Can you work these out from the drawing? Everything is in mm from the part's minimum corner. A direction names the side the tool comes from. Give positions to 0.01 mm unless a question says otherwise; leave off trailing zeros. Order: outer loops, then holes, each group sorted by start corner. A loop starts at its lowest first (then second) coordinate and runs counter-clockwise, first axis right, second up. Notation, with made-up numbers: (-28, 19) - (11, 19) arc R23 ccw to (11, 29) - close; hole circle Ø5 at (82.5, 30.5). An arc over 180 degrees is marked (long way). Answer as a JSON object with one key per item and string values.
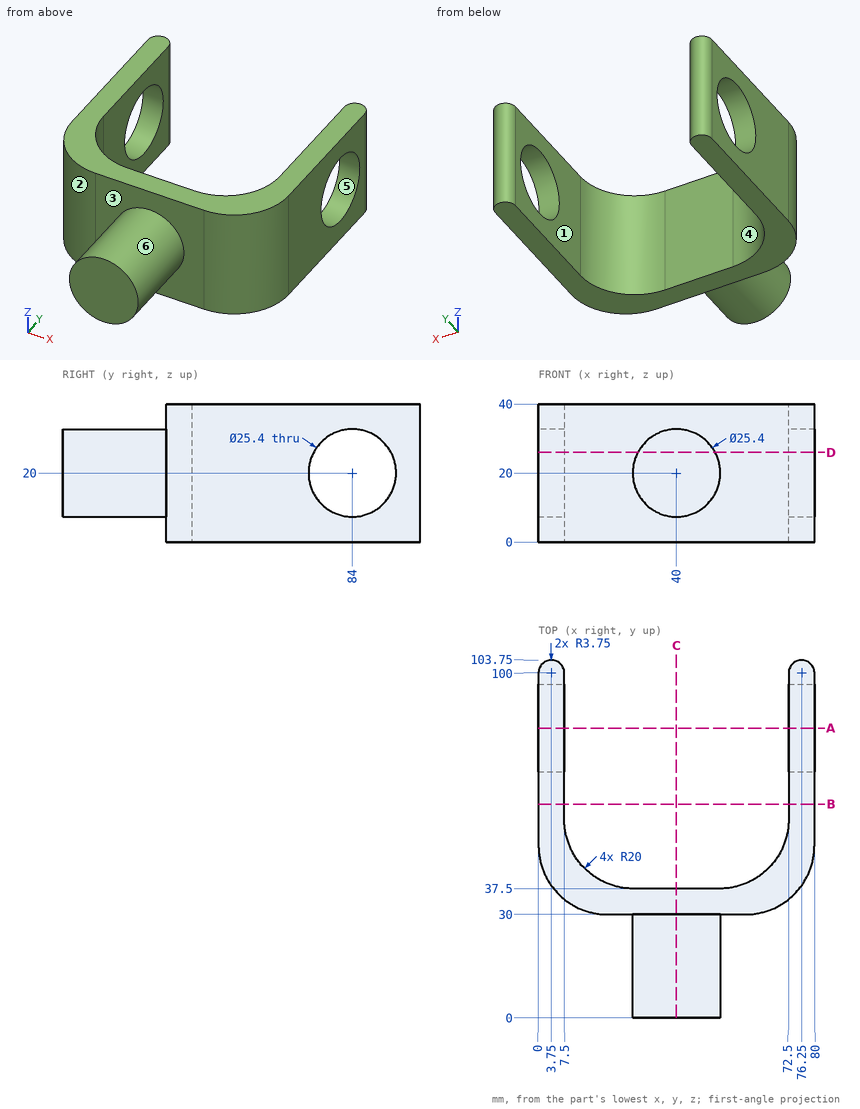
Q1. I'm going to push flat-ended pins straight in: pin 1 Ø4 at (x, z) = (58.5, 26) entering from +Y; pin 2 Ø5 at (x, z) = (59, 23.5) entering from -Y; pin 3 Ø1 at (x, z) = (34.5, 27.5) entering from +Y. Where does each tip first touch, or does it pass through?
Recorded:
{"pin 1": "stops at y = 39.17", "pin 2": "stops at y = 30", "pin 3": "stops at y = 37.5"}
Q2. If we section it at C-C, the plane x = 40: Please give me the cut outline in (y, z), then the cut area to 3 significant figures.
Recorded:
{"outline": "(0, 7.3) - (30, 7.3) - (30, 0) - (37.5, 0) - (37.5, 40) - (30, 40) - (30, 32.7) - (0, 32.7) - close", "area": "1,060 mm^2"}
Q3. We'd pull the mould along Z, two halves only. Please class the marked faces 4, 5 and 6: released by +Z, released by -Z, zero draft, split by the parting line, or undercut.
Recorded:
{"face 4": "zero draft", "face 5": "undercut", "face 6": "split by the parting line"}
Q4. If we section it at A-A, the plane y = 84: Please give me the cut outline in (x, z).
Recorded:
{"outline": "(0, 0) - (7.5, 0) - (7.5, 7.3) - (0, 7.3) - close; (0, 32.7) - (7.5, 32.7) - (7.5, 40) - (0, 40) - close; (72.5, 0) - (80, 0) - (80, 7.3) - (72.5, 7.3) - close; (72.5, 32.7) - (80, 32.7) - (80, 40) - (72.5, 40) - close"}
Q5. If we section it at D-D, the plane z = 26: Please give me the cut outline in (x, y).
Recorded:
{"outline": "(0, 50) arc R20 ccw to (20, 30) - (28.81, 30) - (28.81, 0) - (51.19, 0) - (51.19, 30) - (60, 30) arc R20 ccw to (80, 50) - (80, 72.81) - (72.5, 72.81) - (72.5, 57.5) arc R20 cw to (52.5, 37.5) - (27.5, 37.5) arc R20 cw to (7.5, 57.5) - (7.5, 72.81) - (0, 72.81) - close; (0, 95.19) - (7.5, 95.19) - (7.5, 100) arc R3.75 ccw to (0, 100) - close; (72.5, 95.19) - (80, 95.19) - (80, 100) arc R3.75 ccw to (72.5, 100) - close"}
Q6. I need wall thicknesses on L1, parallel to Z at x = 2.75, y = 84; L2, parallel to X at y = 70, z = 26.5; L3, parallel to Y at x = 77, z = 20. Which ranges of each line are inside material? Lowest first, please.
Recorded:
{"L1": "z = 0 to 7.3, 32.7 to 40", "L2": "x = 0 to 7.5, 72.5 to 80", "L3": "y = 39.46 to 71.3, 96.7 to 103.67"}
Q7. Which directions (+Z, -Z, +X, -X, +Y, -Y) give clear straight access to the entire face, cutting with the end or side of a thin tool? Please do the marked faces 1, 2 and 3.
Recorded:
{"face 1": "+Z, -Z, +Y", "face 2": "+Z, -Z, -X, -Y", "face 3": "-Y"}
Q8. If we section it at B-B, the plane y = 62: Please give me the cut outline in (x, z), then the cut area to 3 significant figures.
Recorded:
{"outline": "(0, 0) - (7.5, 0) - (7.5, 40) - (0, 40) - close; (72.5, 0) - (80, 0) - (80, 40) - (72.5, 40) - close", "area": "600 mm^2"}
